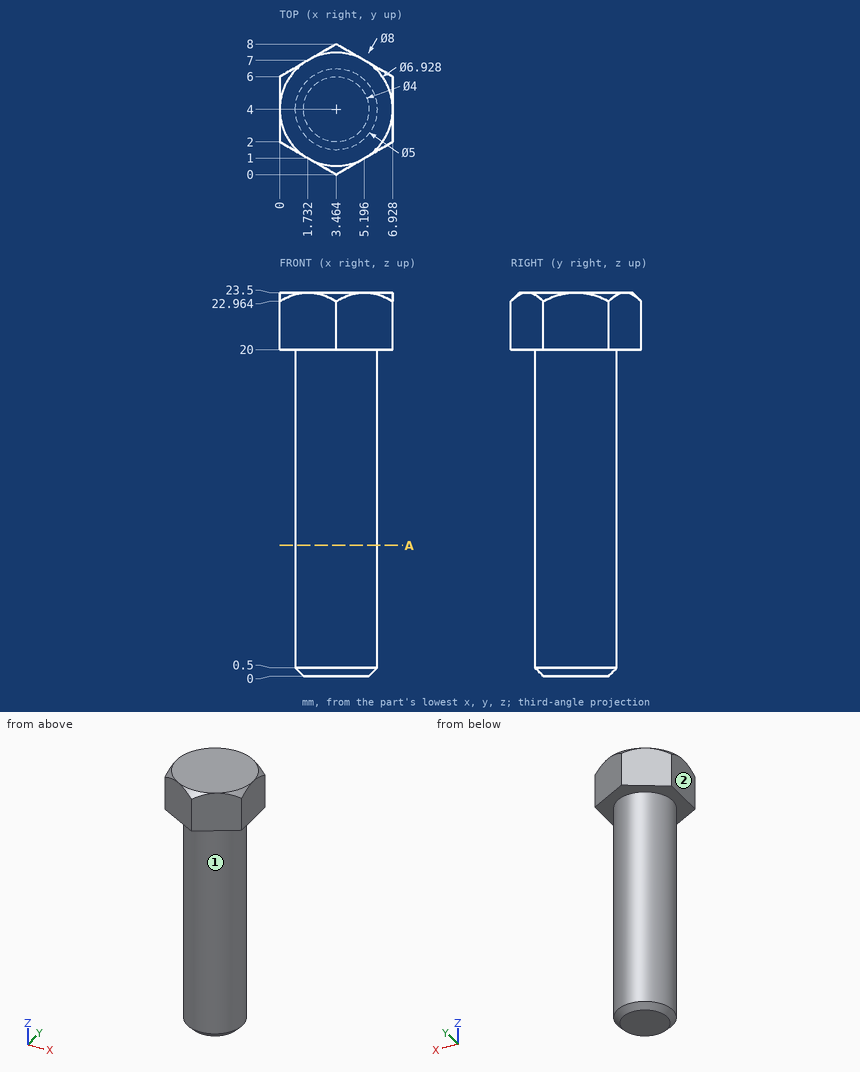
Study the drawing (mm; zero at the part's minimum x, y, z) and answer. A direction names the side the tool comes from. Coordinates: 2 decimals unless noted, no trailing zeros. Loops run counter-clockwise (first coordinate to the right, second up) from the corner with the lowest first, then second, coordinate; pieces in that order, holes last. Notation, with made-up numbers: M 20.5,52.5 L 49.5,52.5 A4 ccw 49.5,59.5 Z; hole C 83,75.5 d11. An arc over 180 degrees is marked long. Answer in a Markdown table with one row per item.
1) Given pin 1 (2 mm diameter, centred on x = 1.5, z = 5, fed in from +Y); pin 2 (2 mm diameter, centred on x = 4.5, y = 5, fed in from -Z); pin 3 (3 mm diameter, centred on x = 5, z = 17, fed in from -Y), each flat-ended and moving along its own axis, determine where each tip first touches the part or whether it passes through.
Answers below:
| item | result |
|---|---|
| pin 1 | y = 6.31 |
| pin 2 | z = 0 |
| pin 3 | y = 1.5 |
2) Which of the six approach directions +Z, -Z, +X, -X, +Y, -Y give full straight-line access (tool end or side, diameter ignored) to the marked faces 1 and 2?
Answers below:
| item | result |
|---|---|
| face 1 | -Z |
| face 2 | +Z, -Z, -X, +Y, -Y |
3) Find the intervals of material crossed by probe 1 along X at (y, z) = (5.5, 13.25) (1 decimal); probe 2 along Z at (x, y) = (2, 6.75); probe 3 along X at (y, z) = (5, 19.25) (1 decimal), in increasing order.
Answers below:
| item | result |
|---|---|
| probe 1 | 1.5 to 5.5 |
| probe 2 | 20 to 23.5 |
| probe 3 | 1.2 to 5.8 |
4) Find section A-A (z = 8). Determine the outline of the cut face in (x, y), then the cut area to 3 significant figures.
Answers below:
| item | result |
|---|---|
| outline | C 3.46,4 d5 |
| area | 19.6 mm^2 |
